Answer from the drawing. Dimensions are ordinates in mm from the lowest x, y and z of the part. A direction names the side the tool comes from. Round coordinates to 2 decimals unless told otherwise and drop trailing zeros. Write each loop counter-clockwise with the first axis right and the second up, starting at its lowest first coordinate (ties: lowest second). Pieces come first, ordered by that corner, then holes. Notation, with made-up numbers: (-8, 82) - (17, 82) arc R5 ccw to (17, 86) - close; hole circle Ø9 at (28, 11.5). An arc over 180 degrees is marked (long way). Use a Markdown table: item, result. Add a question column.
1) A cutting plane is placed at D-D (x = 77). Give the vertices of the cut face in (y, z), then the cut area to 3 significant figures.
2) Find the intervals of material crossed by probe 1 along Z at (x, y) = (77, 1.25); probe 2 along X at (y, z) = (0.95, 3); probe 3 along Y at (x, z) = (5, 39.5), in increasing order. Write a range as from..to.
3) A cutting plane is placed at A-A (z = 20). Give the vertices of the cut face in (x, y), then the cut area to 3 significant figures.
4) A tool of negligible diameter and unlimited length cuts with its end or side. For the marked faces 1 and 2, from which of +Z, -Z, +X, -X, +Y, -Y can it reach the whole face along a straight path? Write none if from no direction.
5) Each of these flat-tipped pins is pushed along its axis until it touches: P1, Ø1.5, axis at x = 9.5, y = 12.5, coming from the -Z side; P2, Ø5, axis at x = 77, z = 3, coming from the +Y side; P3, Ø1.8, axis at x = 3, z = 57, coming from the -Y side. Where does it stop, or does it pass through?
6) A cutting plane is placed at B-B (x = 3). Give the vertices of the cut face in (y, z).
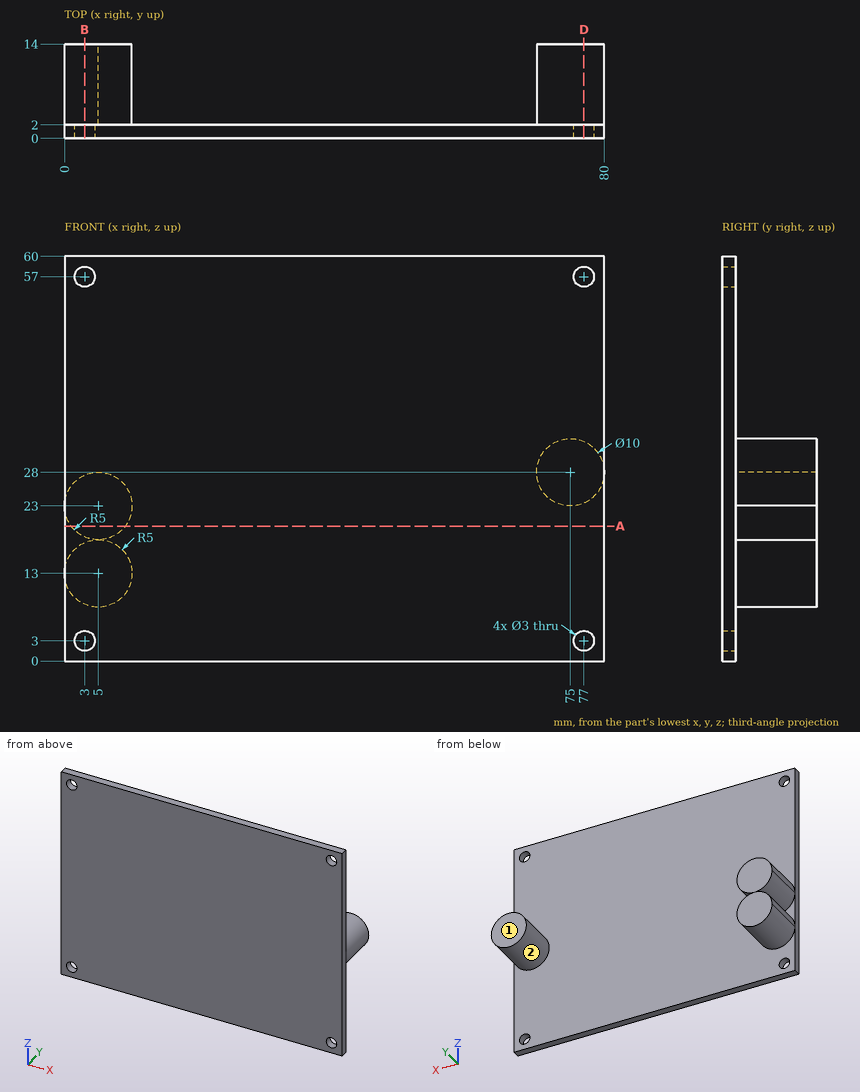
Entries:
| question | item | result |
|---|---|---|
| 1 | outline | (0, 0) - (2, 0) - (2, 1.5) - (0, 1.5) - close; (0, 4.5) - (2, 4.5) - (2, 23.42) - (14, 23.42) - (14, 32.58) - (2, 32.58) - (2, 55.5) - (0, 55.5) - close; (0, 58.5) - (2, 58.5) - (2, 60) - (0, 60) - close |
| 1 | area | 218 mm² |
| 2 | probe 1 | z = 0..1.5, 4.5..55.5, 58.5..60 |
| 2 | probe 2 | x = 0..1.5, 4.5..75.5, 78.5..80 |
| 2 | probe 3 | y = 0..2 |
| 3 | outline | (0, 0) - (80, 0) - (80, 2) - (9, 2) - (9, 14) - (1, 14) - (1, 2) - (0, 2) - close |
| 3 | area | 256 mm² |
| 4 | face 1 | +Z, -Z, +X, -X, +Y |
| 4 | face 2 | +Y |
| 5 | P1 | stops at z = 9.69 |
| 5 | P2 | stops at y = 2 |
| 5 | P3 | passes through |
| 6 | outline | (0, 0) - (2, 0) - (2, 1.5) - (0, 1.5) - close; (0, 4.5) - (2, 4.5) - (2, 8.42) - (14, 8.42) - (14, 17.58) - (2, 17.58) - (2, 18.42) - (14, 18.42) - (14, 27.58) - (2, 27.58) - (2, 55.5) - (0, 55.5) - close; (0, 58.5) - (2, 58.5) - (2, 60) - (0, 60) - close |
